```python
from build123d import *

# Parameters (mm, degrees)
F1_DEPTH = 5.588
F2_R     = 5.08
F3_R     = 5.08


with BuildPart() as f1:
    # F0 (on Front) → F1 (new body, symmetric)
    with BuildSketch(Plane.XZ):
        with BuildLine():
            Line((-24.003, -32.512), (24.003, -32.512))
            Line((24.003, -32.512), (24.003, 26.162))
            ThreePointArc((24.003, 26.162), (22.1431280605, 30.6521280605), (17.653, 32.512))
            Line((17.653, 32.512), (-17.653, 32.512))
            ThreePointArc((-17.653, 32.512), (-22.1431280605, 30.6521280605), (-24.003, 26.162))
            Line((-24.003, 26.162), (-24.003, -32.512))
        make_face()
    extrude(amount=F1_DEPTH, both=True)

    # F2
    f2_edges = [f1.edges().sort_by_distance(p)[0] for p in [
        (-22.143128, 5.588, 30.652128),
        (-24.003, 0, 26.162),
        (-22.143128, -5.588, 30.652128),
        (-17.653, 0, 32.512),
    ]]
    fillet(f2_edges, radius=F2_R)

    # F3
    f3_edges = [f1.edges().sort_by_distance(p)[0] for p in [
        (-22.515102, -4.100102, -32.512),
        (22.515102, -4.100102, -32.512),
    ]]
    fillet(f3_edges, radius=F3_R)


solid = f1.part
```
Check sheet for the modelled part. Datum: model origin and axes. Units: mm. Round coordinates to 2 decimals unless told otherwise and drop trailing zeros. Order: outer loops, then holes, each group sorted by start corner. A loop starts at its lowest first (then second) coordinate and runs counter-clockwise, first axis right, second up.
1) Scan lines: line 1 (Z direction, x = 18, y = -0.5); line 2 (Z direction, x = 1, y = -4.75); line 3 (Y direction, x = 4.5, z = 28). Record each from-to range of solid material in increasing order.
2) Go/stop test with flat-tipped pins: pin 1 Ø1 at (x, y) = (-17.5, -2) entering from -Z; pin 2 Ø4 at (y, z) = (-4, 3) entering from -X. Record where each tip stops, or that it passes through.
3) Section check B-B (z = 23). Record the boundary of the cut face in (x, y), and give its area (3 significant figures).
4) Section check A-A (x = 6). Record the boundary of the cut face in (y, z), and give its area (3 significant figures).
Result:
1. line 1: z = -32.51 to 32.5
1. line 2: z = -30.23 to 30.23
1. line 3: y = -5.56 to 5.56
2. pin 1: stops at z = -32.41
2. pin 2: stops at x = -23.78
3. outline: (-24, -0.51) arc R5.08 ccw to (-18.92, -5.59) - (18.92, -5.59) arc R5.08 ccw to (24, -0.51) - (24, 0.51) arc R5.08 ccw to (18.92, 5.59) - (-18.92, 5.59) arc R5.08 ccw to (-24, 0.51) - close
3. area: 514 mm2
4. outline: (-5.59, -27.43) arc R5.08 ccw to (-0.51, -32.51) - (0.51, -32.51) arc R5.08 ccw to (5.59, -27.43) - (5.59, 27.43) arc R5.08 ccw to (0.51, 32.51) - (-0.51, 32.51) arc R5.08 ccw to (-5.59, 27.43) - close
4. area: 705 mm2
